Geometry check sheet. Reference: drawing and pictorial views, mm from the part's lowest x, y, z. A direction names the side the tool comes from. Round coordinates to 2 decimals unless told otherwise and drop trailing zeros. Order: outer loops, then holes, each group sorted by start corner. A loop starts at its lowest first (then second) coordinate and runs counter-clockwise, first axis right, second up. Notation, with made-up numbers: (-17, 33.25) -> (19, 33.25) arc R20 ccw to (19, 46.25) -> close; hole circle Ø11 at (34, 83.5). An arc over 180 degrees is marked (long way). Return JSON: item names as keys, results as strings. Group by question number.
1) Scan lines: L1, parallel to Y at x = 19.05, z = 2.45; L2, parallel to Z at x = 21.5, y = 54.5 (1 decimal); L3, parallel to X at y = 10, z = 7. Record each from-to range of solid material in increasing order.
2) Tool access check on the marked faces 1, 2 and 3. Record the directions out of +Z, -Z, +X, -X, +Y, -Y that give a thin tool (end or side, any length) a straight path to the whole face; none if there is none.
3) Section check A-A on y = 31.75. State how many separate pieces and enclosed holes the cut face has.
4) Section check D-D on z = 34. Enter the section's corners in (x, y).
5) Depth check by flat-ended pin: pin 1 (6.5 mm diameter, centred on x = 6.35, y = 6.35, fed in from +Z) (3 decimals); pin 2 (3 mm diameter, centred on y = 7, z = 43.5, fed in from +X); pin 3 (4 mm diameter, centred on x = 81.5, y = 36, fed in from -Z). Enter the tip coordinate at first touch or a pass-through.
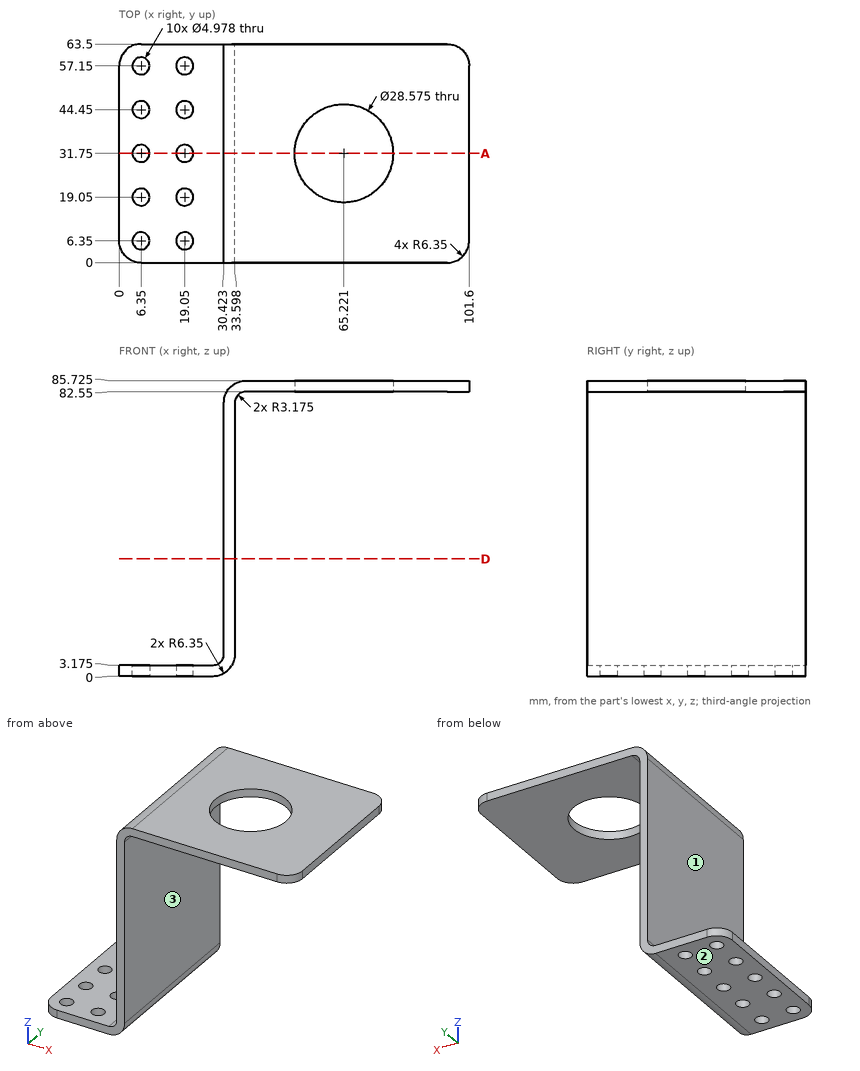
Check result:
{
 "1": {"L1": "0 to 3.86, 8.84 to 16.56, 21.54 to 29.26, 34.24 to 41.96, 46.94 to 54.66, 59.64 to 63.5", "L2": "0 to 3.2", "L3": "30.42 to 33.6"},
 "2": {"face 1": "+Z, -X, +Y, -Y", "face 2": "-Z, +X, -X, +Y, -Y", "face 3": "-Z, +X, +Y, -Y"},
 "3": {"separate pieces": "4", "enclosed holes": "0"},
 "4": {"outline": "(30.42, 0) -> (33.6, 0) -> (33.6, 63.5) -> (30.42, 63.5) -> close"},
 "5": {"pin 1": "z = 3.175", "pin 2": "x = 33.6", "pin 3": "z = 82.55"}
}
